The model under review builds one solid part; all positions refer to its coordinate system, in mm. A direction names the side the tool comes from. Give positions to 0.01 mm unless a question says otherwise; leave off trailing zeros. Order: outer loops, then holes, each group sorted by start corner. A loop starts at its lowest first (then second) coordinate and runs counter-clockwise, first axis right, second up.
```python
from build123d import *

# Parameters (mm, degrees)
SKETCH_W        = 85
SKETCH_H        = 110
PAD_DEPTH       = 3.5
SKETCH001_R     = 0.75
POCKET_DEPTH    = 9
SKETCH002_R     = 3
POCKET001_DEPTH = 2.5
SKETCH003_W     = 85
SKETCH003_H     = 110
PAD001_DEPTH    = 18
SKETCH004_W     = 81
SKETCH004_H     = 106
POCKET002_DEPTH = 18
SKETCH005_R     = 9
SKETCH005_R_2   = 8
SKETCH005_W     = 14
SKETCH005_H     = 11
SKETCH005_W_2   = 12
SKETCH005_H_2   = 10
POCKET003_DEPTH = 5
SKETCH006_W     = 81
SKETCH006_H     = 106
POCKET004_DEPTH = 18
SKETCH007_R     = 8
SKETCH007_W     = 13
SKETCH007_H     = 11
POCKET005_DEPTH = 5
SKETCH008_R     = 2.25
POCKET006_DEPTH = 5
SKETCH009_W     = 83
SKETCH009_H     = 108
POCKET007_DEPTH = 2.5
SKETCH010_R     = 6.5
POCKET008_DEPTH = 5


with BuildPart() as part:
    # Sketch → Pad (new body)
    with BuildSketch(Plane.XY):
        Rectangle(SKETCH_W, SKETCH_H)
    extrude(amount=PAD_DEPTH)

    # Sketch001 (on Face6 of Pad) → Pocket (cut)
    with BuildSketch(Plane.XY.offset(3.5)):
        with Locations((-24.13, -27.5)):
            Circle(SKETCH001_R)
        with Locations((24.13, -28.96)):
            Circle(SKETCH001_R)
        with Locations((-8.89, 23.11)):
            Circle(SKETCH001_R)
    extrude(amount=-POCKET_DEPTH, mode=Mode.SUBTRACT)

    # Sketch002 (on Face4 of Pocket) → Pocket001 (cut)
    with BuildSketch(Plane(origin=(0, 0, 0), x_dir=(1, 0, 0), z_dir=(0, 0, -1))):
        with Locations((-8.89, -23.11)):
            Circle(SKETCH002_R)
        with Locations((-24.13, 27.5)):
            Circle(SKETCH002_R)
        with Locations((24.13, 28.96)):
            Circle(SKETCH002_R)
    extrude(amount=-POCKET001_DEPTH, mode=Mode.SUBTRACT)

    # Sketch003 (on Face5 of Pocket001) → Pad001 (join)
    with BuildSketch(Plane.XY.offset(3.5)):
        Rectangle(SKETCH003_W, SKETCH003_H)
    extrude(amount=PAD001_DEPTH)

    # Sketch004 (on Face12 of Pad001) → Pocket002 (cut)
    with BuildSketch(Plane.XY.offset(21.5)):
        Rectangle(SKETCH004_W, SKETCH004_H)
    extrude(amount=-POCKET002_DEPTH, mode=Mode.SUBTRACT)

    # Sketch005 (on Face13 of Pocket002) → Pocket003 (cut)
    with BuildSketch(Plane.XZ.offset(55)):
        with Locations((-12.67, 19.5)):
            Circle(SKETCH005_R)
        with Locations((10.303566, 33.5)):
            Circle(SKETCH005_R_2)
        with Locations((18.67, 16)):
            Rectangle(SKETCH005_W, SKETCH005_H)
        with Locations((21.67, 28.5)):
            Rectangle(SKETCH005_W_2, SKETCH005_H_2)
    extrude(amount=-POCKET003_DEPTH, mode=Mode.SUBTRACT)

    # Sketch006 (on Face12 of Pocket003) → Pocket004 (cut)
    with BuildSketch(Plane.XY.offset(21.5)):
        Rectangle(SKETCH006_W, SKETCH006_H)
    extrude(amount=-POCKET004_DEPTH, mode=Mode.SUBTRACT)

    # Sketch007 (on Face5 of Pocket004) → Pocket005 (cut)
    with BuildSketch(Plane(origin=(0, 55, 0), x_dir=(-1, 0, 0), z_dir=(0, 1, 0))):
        with Locations((1.33, 21.5)):
            Circle(SKETCH007_R)
        with Locations((-16.17, 16)):
            Rectangle(SKETCH007_W, SKETCH007_H)
    extrude(amount=-POCKET005_DEPTH, mode=Mode.SUBTRACT)

    # Sketch008 (on Face36 of Pocket005) → Pocket006 (cut)
    with BuildSketch(Plane.XY.offset(3.5)):
        with Locations((-36.21, 48.71)):
            Circle(SKETCH008_R)
        with Locations((36.21, 48.71)):
            Circle(SKETCH008_R)
        with Locations((-36.21, -48.71)):
            Circle(SKETCH008_R)
        with Locations((36.21, -48.71)):
            Circle(SKETCH008_R)
    extrude(amount=-POCKET006_DEPTH, mode=Mode.SUBTRACT)

    # Sketch009 (on Face22 of Pocket006) → Pocket007 (cut)
    with BuildSketch(Plane.XY.offset(21.5)):
        Rectangle(SKETCH009_W, SKETCH009_H)
    extrude(amount=-POCKET007_DEPTH, mode=Mode.SUBTRACT)

    # Sketch010 (on Face24 of Pocket007) → Pocket008 (cut)
    with BuildSketch(Plane.XY.offset(3.5)):
        with Locations((-20, 40)):
            Circle(SKETCH010_R)
    extrude(amount=-POCKET008_DEPTH, mode=Mode.SUBTRACT)


solid = part.part
```
Item 1: Clearance check with flat-ended pins moving along their axes: pin 1 Ø11 at (x, z) = (-12.67, 19.5) entering from -Y; pin 2 Ø6 at (x, y) = (31.5, 1) entering from +Z; pin 3 Ø0.5 at (x, y) = (4.5, -53.5) entering from +Z. State where each tip first meets the part, or that it passes through.
Values found:
pin 1: stops at y = 53
pin 2: stops at z = 3.5
pin 3: stops at z = 19
Item 2: Take a section at B-B (x = -1.33). Give the boundary of the cut face in (y, z), and give its area (4 significant figures).
Values found:
outline: (-55, 0) - (55, 0) - (55, 13.5) - (53, 13.5) - (53, 3.5) - (-53, 3.5) - (-53, 19) - (-54, 19) - (-54, 21.5) - (-55, 21.5) - close
area: 438.5 mm2
Item 3: Take a section at C-C (y = -37.5). Give the boundary of the cut face in (x, z).
Values found:
outline: (-42.5, 0) - (42.5, 0) - (42.5, 21.5) - (41.5, 21.5) - (41.5, 19) - (40.5, 19) - (40.5, 3.5) - (-40.5, 3.5) - (-40.5, 19) - (-41.5, 19) - (-41.5, 21.5) - (-42.5, 21.5) - close
Item 4: For faces 3 (the flat face through (25, -28, 2.5)), 4 (the flat face through (-42, 0, 21.5)), 5 (the flat face through (33, -54, 20)), list the 3-axis set-ups (+Z, -Z, +X, -X, +Y, -Y) from which the entire face can be reached by the end or side of a thin tool; tool diameter is ignored.
Values found:
face 3: -Z
face 4: +Z, +X, -X, +Y, -Y
face 5: +Z
Item 5: Take a section at D-D (x = -31). Give the boundary of the cut face in (y, z), and give its area (3 significant figures).
Values found:
outline: (-55, 0) - (55, 0) - (55, 21.5) - (54, 21.5) - (54, 19) - (53, 19) - (53, 3.5) - (-53, 3.5) - (-53, 19) - (-54, 19) - (-54, 21.5) - (-55, 21.5) - close
area: 452 mm2
Item 6: For line 1 (X direction, y = -18, z = 19.5); line 2 (Y direction, x = -37.5, z = 9.5); line 3 (Y direction, x = -36.21, z = 1.55), list the stretches that pass through material, from the lowest coordinate up.
Values found:
line 1: x = -42.5 to -41.5, 41.5 to 42.5
line 2: y = -55 to -53, 53 to 55
line 3: y = -55 to -50.96, -46.46 to 46.46, 50.96 to 55
Item 7: Draft analysis for pull direction Y (two halves, no side actions). For faces 1 (the cylindrical face through (-9.54, 26.04, 1.23)), 2 (the flat face through (-42.5, -1, 11)), state which applies: released by +Y, released by -Y, zero draft, split by the parting line, or undercut.
Values found:
face 1: undercut
face 2: zero draft
Item 8: Take a section at A-A (y = 40). Give the boundary of the cut face in (x, z), and give its area (3 significant figures).
Values found:
outline: (-42.5, 0) - (-26.5, 0) - (-26.5, 3.5) - (-40.5, 3.5) - (-40.5, 19) - (-41.5, 19) - (-41.5, 21.5) - (-42.5, 21.5) - close; (-13.5, 0) - (42.5, 0) - (42.5, 21.5) - (41.5, 21.5) - (41.5, 19) - (40.5, 19) - (40.5, 3.5) - (-13.5, 3.5) - close
area: 319 mm2
